Check sheet for the modelled part. Datum: model origin and axes. Units: mm. Face numbers are marked on the shaded views. A direction names the side the tool comes from. Give positions to 0.01 mm unless a question says otherwise; leave off trailing zeros. Order: outer loops, then holes, each group sorted by start corner. A loop starts at its lowest first (then second) coordinate and runs counter-clockwise, first axis right, second up. Notation, with made-up numbers: (64, -11) -> (86, -11) arc R4 ccw to (86, -4) -> close; hole circle Ø11 at (47.25, 7). An arc over 180 degrees is marked (long way). One line per question, with ' | ' between items. Start each with the question number.
from build123d import *

# Parameters (mm, degrees)
SKETCH1_W           = 69.85
SKETCH1_H           = 38.1
SKETCH1_R           = 3.175
BOSS_EXTRUDE1_DEPTH = 3.9624
BOSS_EXTRUDE2_DEPTH = 17.4625
BOSS_EXTRUDE4_START = 9.5377
SKETCH1_5_R         = 5.55625
BOSS_EXTRUDE4_DEPTH = 7.9248
BOSS_EXTRUDE5_START = -17.4625
SKETCH1_6_R         = 5.55625
BOSS_EXTRUDE5_DEPTH = 7.9248
FILLET1_R           = 3.81


with BuildPart() as part:
    # Sketch1 → Boss-Extrude1 (new, symmetric)
    # profile 1 of 2: a face of its own
    with BuildSketch(Plane(origin=(0, 0, 0), x_dir=(0, 0, -1), z_dir=(1, 0, 0))):
        with Locations((34.925, -19.05)):
            Rectangle(SKETCH1_W, SKETCH1_H)
        with Locations((16.002, -19.05)):
            Circle(SKETCH1_R, mode=Mode.SUBTRACT)
        with Locations((54.102, -19.05)):
            Circle(SKETCH1_R, mode=Mode.SUBTRACT)
    # profile 2 of 2: a face of its own
    with BuildSketch(Plane(origin=(0, 0, 0), x_dir=(0, 0, -1), z_dir=(1, 0, 0))):
        with BuildLine():
            Line((69.85, -38.1), (0, -38.1))
            ThreePointArc((0, -38.1), (-1.726202144, -43.608432839), (-6.287366834, -47.146565517))
            Line((-6.287366834, -47.146565517), (-20.208052372, -52.324))
            Line((-20.208052372, -52.324), (69.85, -52.324))
            Line((69.85, -52.324), (69.85, -38.1))
        make_face()
    extrude(amount=BOSS_EXTRUDE1_DEPTH, both=True)

    # Sketch1<3> → Boss-Extrude2 (add, symmetric)
    with BuildSketch(Plane(origin=(0, 0, 0), x_dir=(0, 0, -1), z_dir=(1, 0, 0))):
        with BuildLine():
            Line((69.85, -38.1), (0, -38.1))
            ThreePointArc((0, -38.1), (-1.726202144, -43.608432839), (-6.287366834, -47.146565517))
            Line((-6.287366834, -47.146565517), (-20.208052372, -52.324))
            Line((-20.208052372, -52.324), (69.85, -52.324))
            Line((69.85, -52.324), (69.85, -38.1))
        make_face()
    extrude(amount=BOSS_EXTRUDE2_DEPTH, both=True)

    # Sketch1<5> → Boss-Extrude4 (add)
    with BuildSketch(Plane(origin=(0, 0, 0), x_dir=(0, 0, -1), z_dir=(1, 0, 0)).offset(BOSS_EXTRUDE4_START)):
        with BuildLine():
            Line((69.85, -60.452), (69.85, -52.324))
            Line((69.85, -52.324), (-20.208052372, -52.324))
            Line((-20.208052372, -52.324), (-28.448, -55.388632763))
            Line((-28.448, -55.388632763), (-42.047327619, -60.446546582))
            ThreePointArc((-42.047327619, -60.446546582), (-47.953946665, -83.454726113), (-28.448, -97.011367237))
            Line((-28.448, -97.011367237), (69.85, -60.452))
        make_face()
        with Locations((-28.448, -76.2)):
            Circle(SKETCH1_5_R, mode=Mode.SUBTRACT)
    extrude(amount=BOSS_EXTRUDE4_DEPTH)

    # Sketch1<6> → Boss-Extrude5 (add)
    with BuildSketch(Plane(origin=(0, 0, 0), x_dir=(0, 0, -1), z_dir=(1, 0, 0)).offset(BOSS_EXTRUDE5_START)):
        with BuildLine():
            Line((69.85, -60.452), (69.85, -52.324))
            Line((69.85, -52.324), (-20.208052372, -52.324))
            Line((-20.208052372, -52.324), (-28.448, -55.388632763))
            Line((-28.448, -55.388632763), (-42.047327619, -60.446546582))
            ThreePointArc((-42.047327619, -60.446546582), (-47.953946665, -83.454726113), (-28.448, -97.011367237))
            Line((-28.448, -97.011367237), (69.85, -60.452))
        make_face()
        with Locations((-28.448, -76.2)):
            Circle(SKETCH1_6_R, mode=Mode.SUBTRACT)
    extrude(amount=BOSS_EXTRUDE5_DEPTH)

    # Fillet1
    # the kernel refuses this fillet: 3.81 mm, written as the material it adds along each edge
    with BuildSketch(Plane(origin=(-3.9624, -38.1, -69.85), x_dir=(-1, 0, 0), z_dir=(0, 0, 1))) as fillet1_piece_1:
        with BuildLine():
            CenterArc((FILLET1_R, -FILLET1_R), FILLET1_R, 90, 90)
            Line((0, -FILLET1_R), (0, 0))
            Line((0, 0), (FILLET1_R, 0))
        make_face()
    extrude(amount=69.85)
    with BuildSketch(Plane(origin=(3.9624, -38.1, -69.85), x_dir=(1, 0, 0), z_dir=(0, 0, 1))) as fillet1_piece_2:
        with BuildLine():
            CenterArc((FILLET1_R, FILLET1_R), FILLET1_R, 180, 90)
            Line((0, FILLET1_R), (0, 0))
            Line((0, 0), (FILLET1_R, 0))
        make_face()
    extrude(amount=69.85)


solid = part.part
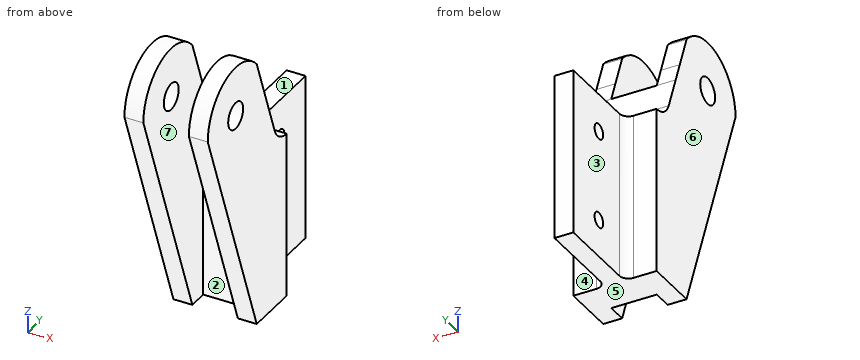
1. Cross-section at B-B on y = -19.05. Record the boundary of the cut face in (x, z).
2. Cross-section at C-C on y = -76.2. Record the boundary of the cut face in (x, z), and give its area (3 significant figures).
3. Tool access check on the marked faces 1, 2, 3 and 4. Record the directions out of +Z, -Z, +X, -X, +Y, -Y that give a thin tool (end or side, any length) a straight path to the whole face; none if there is none.
4. Cross-section at A-A on x = 15.5. Record the boundary of the cut face in (y, z), and give its area (3 significant figures).
5. Cross-section at D-D on z = -10. Record the boundary of the cut face in (x, y).
6. Scan lines: probe 1 along X at (y, z) = (-80.5, 4); probe 2 along Y at (x, z) = (-7.5, -10.5); probe 3 along X at (y, z) = (-8.5, -19). Record each from-to range of solid material in increasing order.
7. Mould release check, pull along X, two halves, no side actions. Record for the marked faces 5, 6 and 7: +X half, -X half, draft (parallel to the pull), parting line (faces both ways), or undercut.
8. Go/stop test with flat-tipped pins: pin 1 (3 mm diameter, centred on x = -14, z = -48, fed in from +Y); pin 2 (8 mm diameter, centred on x = 12, z = -1.5, fed in from -Y); pin 3 (8 mm diameter, centred on x = -12, z = 8, fed in from -Y). Record where each tip stops, or that it passes through.
Response values:
1) outline: (-3.96, -69.85) -> (3.96, -69.85) -> (3.96, -57.28) -> (-3.96, -57.28) -> close; (-3.96, -50.93) -> (3.96, -50.93) -> (3.96, -19.18) -> (-3.96, -19.18) -> close; (-3.96, -12.83) -> (3.96, -12.83) -> (3.96, 0) -> (-3.96, 0) -> close
2) outline: (-17.46, -27.51) -> (-9.54, -27.51) -> (-9.54, 22.89) -> (-17.46, 22.89) -> close; (-17.46, 34) -> (-9.54, 34) -> (-9.54, 49.26) -> (-17.46, 49.26) -> close; (9.54, -27.51) -> (17.46, -27.51) -> (17.46, 22.89) -> (9.54, 22.89) -> close; (9.54, 34) -> (17.46, 34) -> (17.46, 49.26) -> (9.54, 49.26) -> close | area: 1,040 mm²
3) face 1: +Z, +X, -X, +Y | face 2: +Z, -Z, -Y | face 3: +Z, -Z, -X, +Y | face 4: +Z, -Z, +X, +Y
4) outline: (-97.01, 28.45) -> (-60.45, -69.85) -> (-38.1, -69.85) -> (-38.1, 0) arc R9.65 cw to (-47.15, 6.29) -> (-60.45, 42.05) arc R20.81 ccw to start; hole circle Ø11.11 at (-76.2, 28.45) | area: 4,230 mm²
5) outline: (-17.46, -82.71) -> (-9.54, -82.71) -> (-9.54, -52.32) -> (9.54, -52.32) -> (9.54, -82.71) -> (17.46, -82.71) -> (17.46, -38.1) -> (7.77, -38.1) arc R3.81 cw to (3.96, -34.29) -> (3.96, 0) -> (-3.96, 0) -> (-3.96, -34.29) arc R3.81 cw to (-7.77, -38.1) -> (-17.46, -38.1) -> close
6) probe 1: x = -17.46 to -9.54, 9.54 to 17.46 | probe 2: y = -52.32 to -38.09 | probe 3: x = -3.96 to 3.96
7) face 5: draft | face 6: -X half | face 7: undercut
8) pin 1: stops at y = -38.1 | pin 2: stops at y = -87.36 | pin 3: stops at y = -90.89
